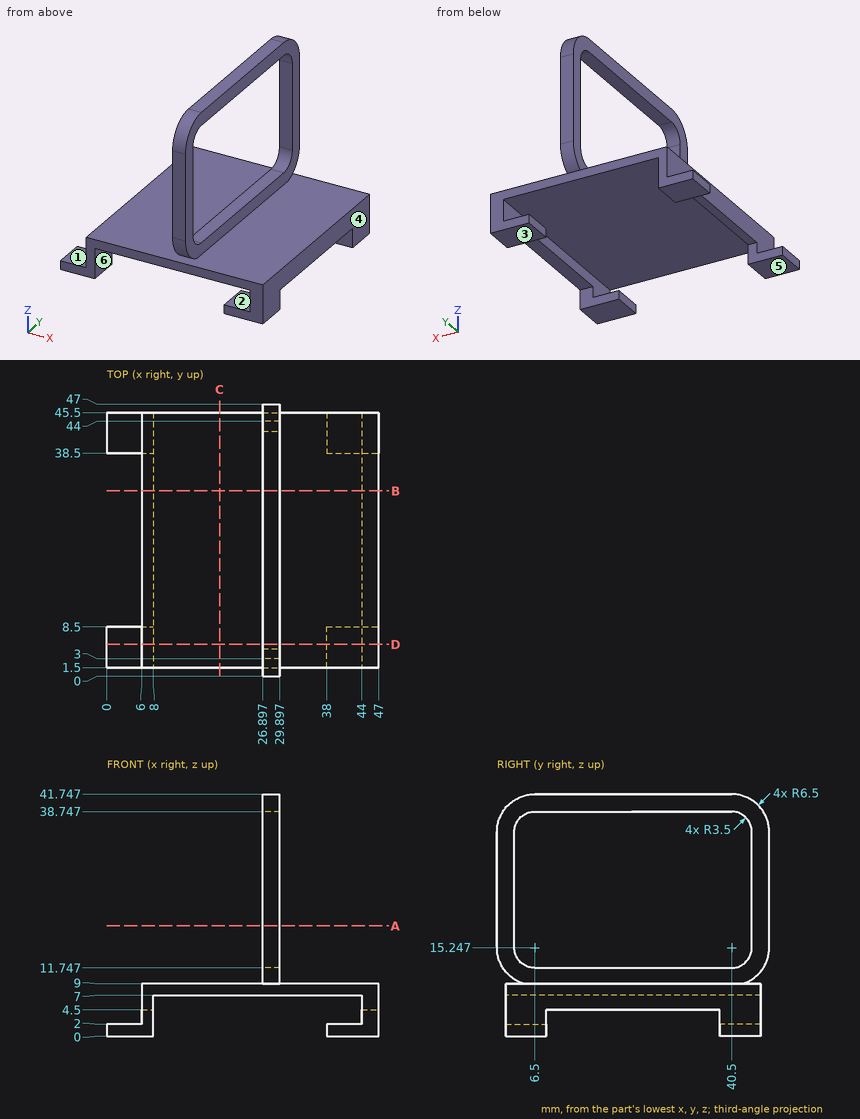
For this review, use the dimensioned drawing (mm, ordinates from the lowest corner) and the shaded views. A direction names the side the tool comes from. Give positions to 0.01 mm unless a question says otherwise; leave off trailing zeros. Order: outer loops, then holes, each group sorted by start corner. A loop starts at its lowest first (then second) coordinate and runs counter-clockwise, first axis right, second up.
1. Mouldability with a two-part tool opening along X and no side actions: class the marked faces 4, 5 and 6 as +X half, -X half, draft (parallel to the pull), parting line (faces both ways), or undercut.
Solution:
face 4: +X half
face 5: draft
face 6: undercut
2. For pin 1 Ø1 at (y, z) = (36, 11) entering from +X; pin 2 Ø1.8 at (x, y) = (4.5, 41.5) entering from +Z; pin 3 Ø1.3 at (x, z) = (41, 2) entering from +Y, all flat-tipped, find the tip position at first contact; note any pin that passes through.
Solution:
pin 1: stops at x = 29.9
pin 2: stops at z = 2
pin 3: stops at y = 45.5
3. Add section A-A, the plane z = 19. State the section outline as (x, y) points, then the cut area to 3 significant figures.
Solution:
outline: (26.9, 0) - (29.9, 0) - (29.9, 3) - (26.9, 3) - close; (26.9, 44) - (29.9, 44) - (29.9, 47) - (26.9, 47) - close
area: 18.0 mm2
4. Add section D-D, the plane y = 5.5. State the section outline as (x, z) points, then the cut area to 3 significant figures.
Solution:
outline: (0, 0) - (8, 0) - (8, 7) - (44, 7) - (44, 2) - (38, 2) - (38, 0) - (47, 0) - (47, 9) - (29.9, 9) - (29.9, 11.89) - (26.9, 11.89) - (26.9, 9) - (6, 9) - (6, 2) - (0, 2) - close; (26.9, 38.6) - (29.9, 38.6) - (29.9, 41.67) - (26.9, 41.67) - close
area: 159 mm2
5. Tool access review of the marked faces 1, 2 and 3: name each direction out of +Z, -Z, +X, -X, +Y, -Y from which nothing blocks a thin tool from reaching the whole face with its end or side.
Solution:
face 1: +Z, -X, +Y, -Y
face 2: +Y, -Y
face 3: -Z, +X, -X, +Y, -Y
6. To check wall thickness, follow L1, parallel to Z at x = 27, y = 22.5; L2, parallel to Y at x = 28, z = 21; L3, parallel to X at y = 34, z = 5.5. State the ranges of each line that lie inside material, in increasing order.
Solution:
L1: z = 7 to 11.75, 38.75 to 41.75
L2: y = 0 to 3, 44 to 47
L3: x = 6 to 8, 44 to 47
7. Add section B-B, the plane y = 32. State the section outline as (x, z) points, then the cut area to 3 significant figures.
Solution:
outline: (6, 4.5) - (8, 4.5) - (8, 7) - (44, 7) - (44, 4.5) - (47, 4.5) - (47, 9) - (29.9, 9) - (29.9, 11.75) - (26.9, 11.75) - (26.9, 9) - (6, 9) - close; (26.9, 38.75) - (29.9, 38.75) - (29.9, 41.75) - (26.9, 41.75) - close
area: 112 mm2
8. Add section C-C, the plane x = 19.5. State the section outline as (y, z) points.
Solution:
outline: (1.5, 7) - (45.5, 7) - (45.5, 9) - (1.5, 9) - close
